Input: dimensioned drawing with shaded views. Units: mm. Origin: part minimum x, y, z. A direction names the side the tool comes from. Round coordinates to 2 decimals unless told otherwise and drop trailing zeros. Loops run counter-clockwise (first coordinate to the right, second up) from the corner with the lowest first, then second, coordinate; pieces in that order, holes last.
Item 1: Access query for the marked faces 1 and 2. Directions: +Z, -Z, +X, -X, +Y, -Y. A direction counts if a zero-diameter tool reaches every point of the face in a straight line with its end or side. Return the directions, or none.
Item 2: Section query B-B on x = 21.5. Return loops of the section in (y, z) (1 decimal).
Item 3: First-contact query: P1, Ø12, axis at x = 10.5, z = 32.5, coming from the -Y side; P2, Ø1.9, axis at x = 17, y = 5, coming from the +Z side; P3, Ø3, axis at x = 23.5, y = 13, coming from the -Z side. Flat tips, straight axial feed; report the tip coordinate or a pass-through.
Item 4: Section query A-A on y = 13.75. Return loops of the section in (x, z).
Item 5: Ray query, L1, parallel to X at y = 13.75, z = 55; L2, parallel to Y at x = 20.5, z = 43 (1 decimal); L3, parallel to Z at x = 12.5, y = 2.75. Return the intervals inside material, ascending.
Item 6: Pull-direction query (X, two-part tool) for the marked faces 3, 4 and 5; classes: released by +X, released by -X, zero draft, split by the parting line, or undercut.
Item 7: Section query D-D on y = 2.5. Return loops of the section in (x, z).
Item 8: Section query C-C on z = 39.5. Return loops of the section in (x, y) (1 decimal).
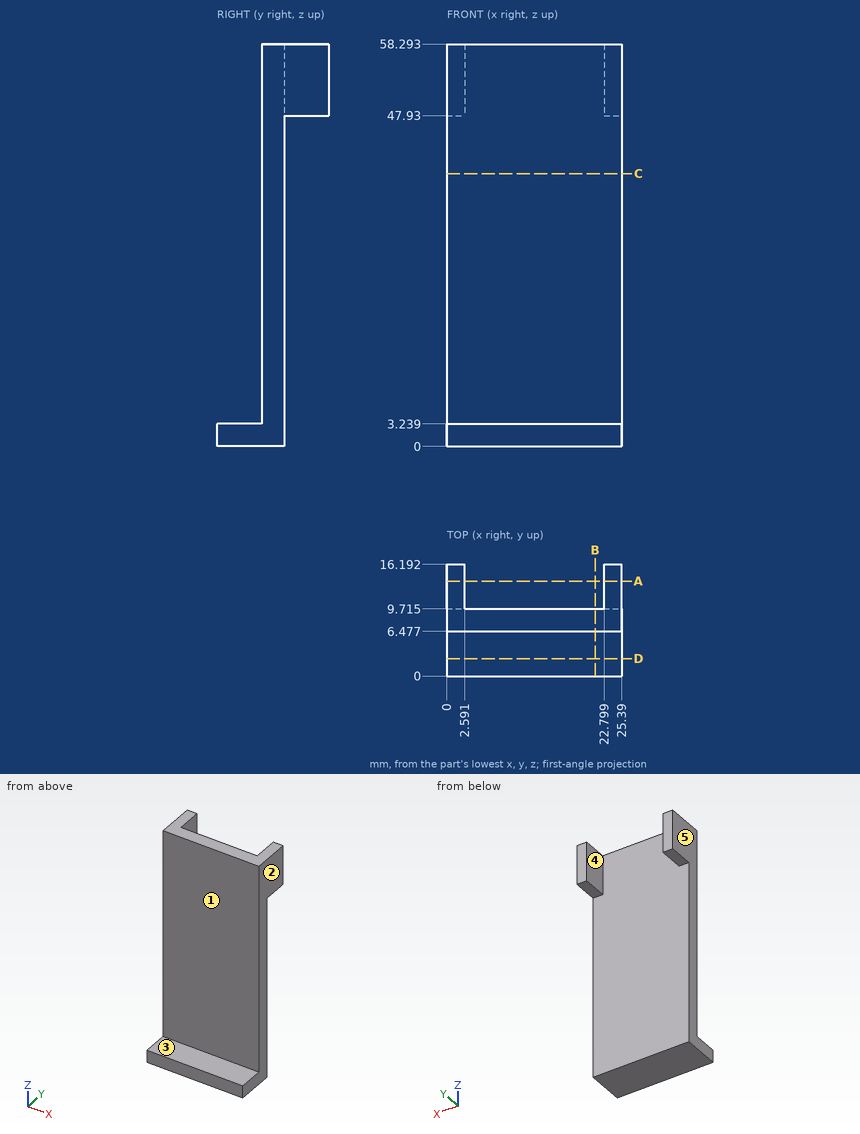
Data:
1. face 1: +Z, +X, -X, -Y
1. face 2: +Z, -Z, +X, +Y, -Y
2. outline: (0, 0) - (9.7, 0) - (9.7, 58.3) - (6.5, 58.3) - (6.5, 3.2) - (0, 3.2) - close
3. P1: stops at y = 6.48
3. P2: stops at z = 3.24
3. P3: stops at z = 47.93
4. outline: (0, 47.93) - (2.59, 47.93) - (2.59, 58.29) - (0, 58.29) - close; (22.8, 47.93) - (25.39, 47.93) - (25.39, 58.29) - (22.8, 58.29) - close
5. L1: x = 0 to 2.59, 22.8 to 25.39
5. L2: y = 6.5 to 9.7
5. L3: z = 0 to 3.24
6. face 3: zero draft
6. face 4: undercut
6. face 5: released by -X
7. outline: (0, 0) - (25.39, 0) - (25.39, 3.24) - (0, 3.24) - close
8. outline: (0, 6.5) - (25.4, 6.5) - (25.4, 9.7) - (0, 9.7) - close
